Verification items for the finished model (mm, model axes). Face numbers are marked on the shaded views. A direction names the side the tool comes from. Coordinates: 2 decimals unless noted, no trailing zeros. Loops run counter-clockwise (first coordinate to the right, second up) from the corner with the lowest first, then second, coordinate; pieces in that order, holes last. Notation, with made-up numbers: (41.25, 60.25) -> (76.25, 60.25) arc R15 cw to (76.25, 79.25) -> close; hole circle Ø8 at (-2, 85.25). An arc over 180 degrees is marked (long way). Write item = value, one per line.
```python
from build123d import *

# Parameters (mm, degrees)
F1_DEPTH    = 10
F2_R        = 3
F3_T1_DEPTH = 81.4336597593


# Not quite as in the source:
# - a fillet or chamfer that OpenCascade refuses, or shapes differently, is made with other operations: its cross-section is extruded or revolved along the edge and cut away or added


with BuildPart() as f1:
    # F0 (on Top) → F1 (new body)
    with BuildSketch(Plane.XY):
        with BuildLine():
            Line((15, 30), (-15, 30))
            Line((-15, 30), (-15, 21.6620222107))
            ThreePointArc((-15, 21.6620222107), (-5, 11.6620222107), (-15, 1.6620222107))
            Line((-15, 1.6620222107), (-15, -30))
            Line((-15, -30), (15, -30))
            Line((15, -30), (15, 1.6620222107))
            ThreePointArc((15, 1.6620222107), (5, 11.6620222107), (15, 21.6620222107))
            Line((15, 21.6620222107), (15, 30))
        make_face()
    extrude(amount=F1_DEPTH)

    # F2
    f2_edges = [f1.edges().sort_by_distance(p)[0] for p in [
        (-5, 11.662022, 10),
        (5, 11.662022, 10),
        (5, 11.662022, 0),
        (-5, 11.662022, 0),
        (0, -30, 0),
        (-15, -14.168989, 0),
        (15, -14.168989, 0),
        (0, -30, 10),
        (15, -14.168989, 10),
        (-15, -14.168989, 10),
        (15, -30, 5),
        (-15, -30, 5),
    ]]
    fillet(f2_edges, radius=F2_R)

    # F3: chamfer of 10 on 1 edges, made by hand

    # F3_s2 → F3_t1 (cut)
    with BuildSketch(Plane.YZ.offset(-40.7168298797)):
        Polygon((20, 10), (30, 0), (30, 10), align=None)
    extrude(amount=F3_T1_DEPTH, mode=Mode.SUBTRACT)


solid = f1.part
```
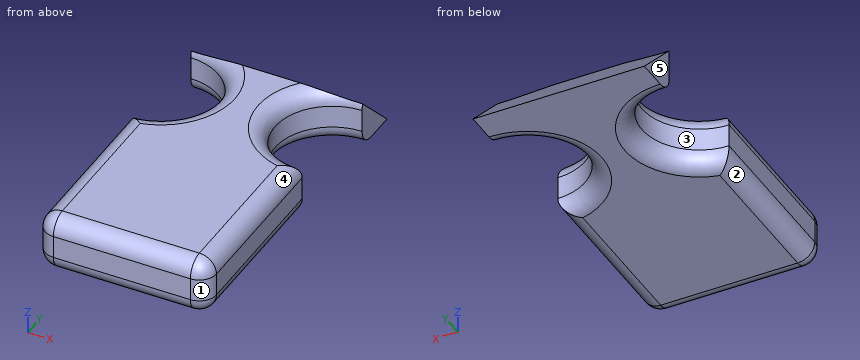
1) Material ranges on line 1 (X direction, y = -14, z = 2.75); line 2 (Y direction, x = -14, z = 3.5); line 3 (Y direction, x = 9, z = 7), recorded low to high.
Ans:
line_1 = -14.99 to 14.99
line_2 = -29.24 to 1.71, 21.61 to 26.5
line_3 = -30 to 3.66, 19.66 to 23
2) Release check for a two-part mould opening along Y. For the marked faces 1, 2 and 3 record: pulls with the +Y half, pulls with the -Y half, needs draft (parallel to the pull), parting line crosses it, or undercut.
Ans:
face_1 = pulls with the -Y half
face_2 = needs draft
face_3 = undercut
3) Depth check by flat-ended pin: pin 1 Ø1 at (y, z) = (3, 5) entering from -X; pin 2 Ø1 at (y, z) = (17.5, 2) entering from -X. Enter the tip coordinate at first touch or a pass-through.
Ans:
pin_1 = -10.99
pin_2 = -7.09
4) Tool access check on the marked faces 4 and 5. Record the directions out of +Z, -Z, +X, -X, +Y, -Y that give a thin tool (end or side, any length) a straight path to the whole face; none if there is none.
Ans:
face_4 = +Z, +X, -Y
face_5 = +Z, -Z, -X, +Y, -Y
5) Sectioned sample at A-A, the plane z = 5.75. Record the cut outline in (x, y).
Ans:
outline = (-15, -27) arc R3 ccw to (-12, -30) -> (12, -30) arc R3 ccw to (15, -27) -> (15, 1.66) arc R10 cw to (15, 21.66) -> (15, 24.25) -> (-15, 24.25) -> (-15, 21.66) arc R10 cw to (-15, 1.66) -> close
6) Sectioned sample at B-B, the plane x = -1. Record the cut outline in (y, z), plus the area to 3 significant figures.
Ans:
outline = (-30, 3) arc R3 ccw to (-27, 0) -> (30, 0) -> (20, 10) -> (-27, 10) arc R3 ccw to (-30, 7) -> close
area = 546 mm2
7) Sectioned sample at C-C, the plane y = -15. Record the cut outline in (x, z).
Ans:
outline = (-15, 3) arc R3 ccw to (-12, 0) -> (12, 0) arc R3 ccw to (15, 3) -> (15, 7) arc R3 ccw to (12, 10) -> (-12, 10) arc R3 ccw to (-15, 7) -> close
